Autodesk Inventor part; units mm, degrees
ref_plane "YZ Plane" through (0, 0, 0) normal (1, 0, 0) x (0, 1, 0)
ref_plane "XZ Plane" through (0, 0, 0) normal (0, 1, 0) x (-1, 0, 0)
ref_plane "XY Plane" through (0, 0, 0) normal (0, 0, 1) x (1, 0, 0)
sketch "Sketch1" plane through (0, 0, 0) normal (0, 0, 1) x (1, 0, 0)
  circle A0 centre (-1.1684, -19.05) radius 2.1844
  circle A1 centre (-1.1684, 19.05) radius 2.1844
  line L0 (3.9688, -24.2345) -> (3.9688, 38.1) construction
  line L1 (-0.0172, -24.9245) -> (-2.3196, -24.9245)
  line L2 (-5.4946, -21.7495) -> (-5.4946, 21.7495)
  line L3 (-2.3196, 24.9245) -> (-0.0172, 24.9245)
  line L4 (3.1578, 21.7495) -> (3.1578, -21.7495)
  line L5 (-2.3196, -24.9245) -> (-5.4946, -21.7495)
  line L6 (-0.0172, -24.9245) -> (3.1578, -21.7495)
  line L7 (-0.0172, 24.9245) -> (3.1578, 21.7495)
  line L8 (-5.4946, 21.7495) -> (-2.3196, 24.9245)
  point P0 (0, 0)
  point P1 (3.1578, -24.9245)
  point P2 (-5.4946, 24.9245)
  point P3 (-5.4946, -24.9245)
  point P4 (3.1578, 24.9245)
  dimension "d0" = 3.175
  dimension "d1" = 3.175
  dimension "d2" = 3.175
  dimension "d3" = 3.175
  dimension "d4" = 3.175
  dimension "d5" = 3.175
  dimension "d6" = 3.175
  dimension "d7" = 3.175
extrude "Extrusion1" add sketch "Sketch1" along normal blind 1.5875
properties part number "Endgame brake pad polycarb"
Input: part model. Units: mm. Frame: model coordinates. Give positions to 0.01 mm unless a question says otherwise; leave off trailing zeros. Write each loop counter-clockwise with the first axis right and the second up, starting at its lowest first coordinate (ties: lowest second). Pieces come first, ordered by that corner, then holes. Notation, with made-up numbers: M -32.5,89.5 L -16.5,89.5 A16 cw -16.5,100.5 Z; hole C -26,15.25 d1. An arc over 180 degrees is marked long. Write item = value, one per line. Start each with the question number.
1) Draft query along Y for faces 1 (the flat face through (-1, 0, 1.588)), 2 (the flat face through (-1, 24.924, 1)), 3 (the cylindrical face through (-1.642, -16.918, 0.783)), 4 (the flat face through (-1, -24.924, 1)). Return one class per face: +Y half, -Y half, draft (parallel to the pull), parting line (faces both ways), or undercut.
2) Cut plane D-D on y = 18. Return the cut outline in (x, z), then the cut area to 3 significant figures.
3) Material intervals for line 1 along Y through (x, z) = (-1, 0.75); line 2 along Y through (x, z) = (0.75, 0.8); line 3 along X through (y, z) = (19, 1.15), sorted ascending. Write a range as [from, to].
4) Cut plane B-B on z = 0.5. Return the cut outline in (x, y), then the cut area to 3 significant figures.
5) Cut plane C-C on x = -1.5. Return the cut outline in (y, z).
6) Cut plane A-A on y = -19.05. Return the cut outline in (x, z), then the cut area to 3 significant figures.
Solved:
q1.face_1 = draft
q1.face_2 = +Y half
q1.face_3 = undercut
q1.face_4 = -Y half
q2.outline = M -5.49,0 L -3.08,0 L -3.08,1.59 L -5.49,1.59 Z; M 0.75,0 L 3.16,0 L 3.16,1.59 L 0.75,1.59 Z
q2.area = 7.65 mm2
q3.line_1 = [-24.92, -21.23], [-16.87, 16.87], [21.23, 24.92]
q3.line_2 = [-24.16, -20.09], [-18.01, 18.01], [20.09, 24.16]
q3.line_3 = [-5.49, -3.35], [1.02, 3.16]
q4.outline = M -5.49,-21.75 L -2.32,-24.92 L -0.02,-24.92 L 3.16,-21.75 L 3.16,21.75 L -0.02,24.92 L -2.32,24.92 L -5.49,21.75 Z; hole C -1.17,-19.05 d4.37; hole C -1.17,19.05 d4.37
q4.area = 381 mm2
q5.outline = M -24.92,0 L -21.21,0 L -21.21,1.59 L -24.92,1.59 Z; M -16.89,0 L 16.89,0 L 16.89,1.59 L -16.89,1.59 Z; M 21.21,0 L 24.92,0 L 24.92,1.59 L 21.21,1.59 Z
q6.outline = M -5.49,0 L -3.35,0 L -3.35,1.59 L -5.49,1.59 Z; M 1.02,0 L 3.16,0 L 3.16,1.59 L 1.02,1.59 Z
q6.area = 6.80 mm2
